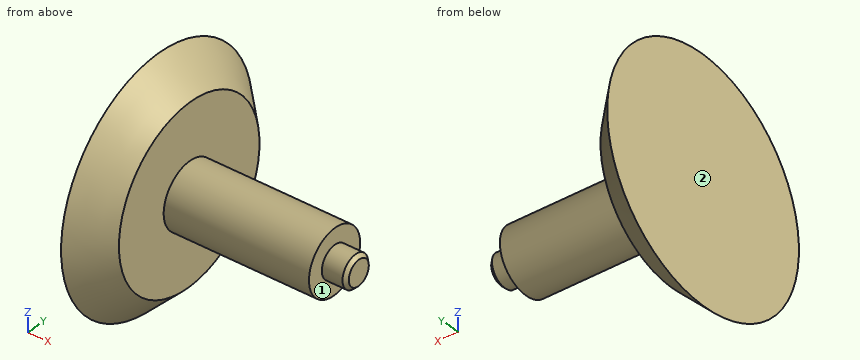
```python
from build123d import *


# Read off the part's stored shape, not the designer's step: M2 机械螺纹 螺柱1
with BuildPart() as part:
    # 草图1 → 旋转1 (revolve)
    with BuildSketch(Plane.XY, mode=Mode.PRIVATE) as revolve_1_sk:
        Polygon((0, 0), (0, 7.5), (2, 5.5), (2, 2), (11, 2), (11, 1), (12.5, 1), (12.5, 0), align=None)
    revolve(revolve_1_sk.sketch.rotate(Axis((0, 0, 0), (1, 0, 0)), 90), axis=Axis((0, 0, 0), (1, 0, 0)))

    # M2 机械螺纹 螺柱1 outline → M2 机械螺纹 螺柱1 (revolve, cut)
    with BuildSketch(Plane.YX):
        Polygon((1, 12.5), (0.7835, 12.5), (1, 12.2835), align=None)
    revolve(axis=Axis((0, 0, 0), (1, 0, 0)), mode=Mode.SUBTRACT)


solid = part.part
```
The model under review builds one solid part; all positions refer to its coordinate system, in mm. Face numbers are marked on the shaded views. A direction names the side the tool comes from. Give positions to 0.01 mm unless a question says otherwise; leave off trailing zeros. Write each loop counter-clockwise with the first axis right and the second up, starting at its lowest first coordinate (ties: lowest second). Pieces come first, ordered by that corner, then holes. Notation, with made-up numbers: (-12, 27.25) -> (8, 27.25) arc R12 ccw to (8, 49.25) -> close; hole circle Ø3 at (-18.5, 25). An arc over 180 degrees is marked (long way). Put each result on its own line as item: value.
(1) We need section C-C, the plane x = 3. Give the boundary of the cut face in (y, z), and give its area (3 significant figures).
Results are:
outline: circle Ø4 at (0, 0)
area: 12.6 mm²
(2) To check wall thickness, follow probe 1 along X at (y, z) = (-1, 5); probe 2 along X at (y, z) = (1.5, -0.75); probe 3 along Y at (x, z) = (6, 0). State the ranges of each line that lie inside material, in increasing order. Write a range as from..to.
Results are:
probe 1: 0..2
probe 2: 0..11
probe 3: -2..2
(3) For pin 1 Ø1.5 at (x, y) = (8.5, 3.5) entering from +Z; pin 2 Ø2 at (y, z) = (-6, 1.5) entering from +X; pin 3 Ø6 at (x, y) = (7.5, 0.5) entering from -Z; pin 4 Ø3.5 at (y, z) = (2.5, -1) entering from +X, all flat-tipped, find the tip position at first contact; note any pin that passes through.
Results are:
pin 1: through
pin 2: x = 2
pin 3: z = -2
pin 4: x = 12.34
(4) Tool access review of the marked faces 1 and 2: name each direction out of +Z, -Z, +X, -X, +Y, -Y from which nothing blocks a thin tool from reaching the whole face with its end or side.
Results are:
face 1: +X
face 2: +Z, -Z, -X, +Y, -Y
(5) We need section A-A, the plane y = 0. Give the boundary of the cut face in (x, z), and give its area (3 significant figures).
Results are:
outline: (0, -7.5) -> (2, -5.5) -> (2, -2) -> (11, -2) -> (11, -1) -> (12.28, -1) -> (12.5, -0.78) -> (12.5, 0.78) -> (12.28, 1) -> (11, 1) -> (11, 2) -> (2, 2) -> (2, 5.5) -> (0, 7.5) -> close
area: 65.0 mm²
